Autodesk Inventor part; units mm, degrees
ref_plane "YZ Plane" through (0, 0, 0) normal (1, 0, 0) x (0, 1, 0)
ref_plane "XZ Plane" through (0, 0, 0) normal (0, 1, 0) x (-1, 0, 0)
ref_plane "XY Plane" through (0, 0, 0) normal (0, 0, 1) x (1, 0, 0)
sketch "Sketch1" plane through (0, 0, 0) normal (0, 0, 1) x (1, 0, 0)
  circle A0 centre (0, 0) radius 38.5
  circle A1 centre (0, 0) radius 40.5
  dimension "Inner_Diameter" = 77
  dimension "d1" = 81
extrude "Extrusion1" add sketch "Sketch1" against normal blind 2 contours A0 | A1
extrude "Extrusion2" add sketch "Sketch1" along normal blind 10
sketch "Sketch2" plane through (0, 0, -2) normal (0, 0, -1) x (-1, 0, 0)
  circle A0 centre (0, 0) radius 2.5
  dimension "Axis_Hole" = 5
extrude "Extrusion3" cut sketch "Sketch2" against normal up to surface (2 mm away) from surface at 0
equation "\"d1\" = Inner_Diameter + 2 * Thickness"
equation "\"Thickness\" = 2"
properties part number "Cap"
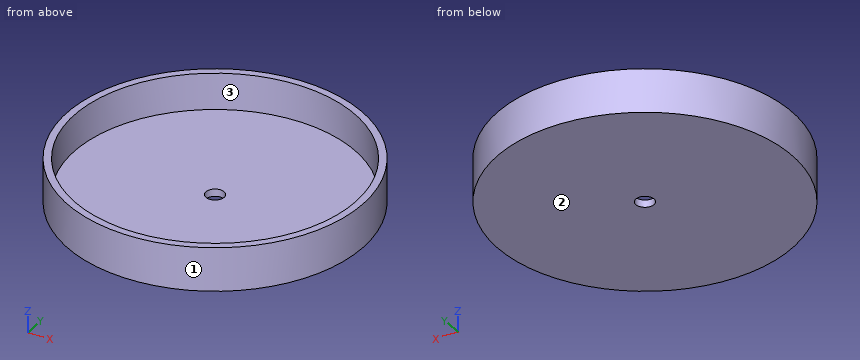
For this review, take the finished solid that the model builds, in its own axes (mm). Face numbers are marked on the shaded views. Round coordinates to 2 decimals unless told otherwise and drop trailing zeros. Write each loop counter-clockwise with the first axis right and the second up, starting at its lowest first coordinate (ties: lowest second). Pieces come first, ordered by that corner, then holes. Notation, with made-up numbers: (23, 5.25) -> (32, 5.25) arc R21 cw to (32, 31.25) -> close; hole circle Ø8 at (-21.5, 46.25). An arc over 180 degrees is marked (long way). One line per question, with ' | ' between items. Start each with the question number.
(1) Add section A-A, the plane y = 0. Write out the cut boundary in (x, z).
(2) Mouldability with a two-part tool opening along X and no side actions: class the marked faces 1, 2 and 3 as released by +X, released by -X, zero draft, split by the parting line, or undercut.
(3) Insertion check: P1, Ø3, axis at x = 4, y = -13.5, coming from the +Z side; P2, Ø1, axis at x = 25.5, z = 8.5, coming from the -Y side; P3, Ø5, axis at y = -10, z = 4, coming from the -X side; P4, Ø4.5, axis at x = 0, y = 0, coming from the -Z side. Each pin has a flat end and moves straight along its axis. Give the tip position at first contact, or say it passes through.
(4) For line 1 along Y through (x, z) = (0, 6.5); line 2 along Y through (x, z) = (0, -1.25); line 3 along Z through (x, y) = (-13, 28), list the stretches that pass through material, from the lowest coordinate up. Write a range as from..to.
(5) Add section C-C, the plane z = 8.75. Write out the cut boundary in (x, y), plus the area to 3 significant figures.
(6) Add section D-D, the plane x = 25.5. Write out the cut boundary in (y, z).
Answer list:
1) outline: (-40.5, -2) -> (-2.5, -2) -> (-2.5, 0) -> (-38.5, 0) -> (-38.5, 10) -> (-40.5, 10) -> close; (2.5, -2) -> (40.5, -2) -> (40.5, 10) -> (38.5, 10) -> (38.5, 0) -> (2.5, 0) -> close
2) face 1: split by the parting line | face 2: zero draft | face 3: undercut
3) P1: z = 0 | P2: y = -31.86 | P3: x = -39.8 | P4: through
4) line 1: -40.5..-38.5, 38.5..40.5 | line 2: -40.5..-2.5, 2.5..40.5 | line 3: -2..0
5) outline: circle Ø81 at (0, 0); hole circle Ø77 at (0, 0) | area: 496 mm²
6) outline: (-31.46, -2) -> (31.46, -2) -> (31.46, 10) -> (28.84, 10) -> (28.84, 0) -> (-28.84, 0) -> (-28.84, 10) -> (-31.46, 10) -> close
